from build123d import *

# Parameters (mm, degrees)
F0_W      = 60
F0_H      = 38
F1_DEPTH  = 2
F2_W      = 55.6
F2_H      = 33.6
F2_W_2    = 53.6
F2_H_2    = 31.6
F3_DEPTH  = 6
F4_W      = 45
F4_H      = 35
F5_DEPTH  = 1
F6_R      = 2
F7_R      = 1
F8_DEPTH  = 8.001
F9_R      = 1
F10_DEPTH = 35.801
F11_SIZE  = 1


with BuildPart() as f1:
    # F0 (on Top) → F1 (new body)
    with BuildSketch(Plane.XY):
        with Locations((30, -19)):
            Rectangle(F0_W, F0_H)
    extrude(amount=F1_DEPTH)

    # F2 (on face) → F3 (join)
    with BuildSketch(Plane.XY.offset(2)):
        with Locations((30, -19)):
            Rectangle(F2_W, F2_H)
        with Locations((30, -19)):
            Rectangle(F2_W_2, F2_H_2, mode=Mode.SUBTRACT)
    extrude(amount=F3_DEPTH)

    # F4 (on face) → F5 (cut)
    with BuildSketch(Plane(origin=(0, 0, 0), x_dir=(1, 0, 0), z_dir=(0, 0, -1))):
        with Locations((24.5, 19)):
            Rectangle(F4_W, F4_H)
    extrude(amount=-F5_DEPTH, mode=Mode.SUBTRACT)

    # F6
    f6_edges = [f1.edges().sort_by_distance(p)[0] for p in [
        (0, -38, 1),
        (0, 0, 1),
        (60, -38, 1),
        (60, 0, 1),
    ]]
    fillet(f6_edges, radius=F6_R)

    # F7 (on face) → F8 (cut, through all)
    with BuildSketch(Plane(origin=(0, 0, 0), x_dir=(1, 0, 0), z_dir=(0, 0, -1))):
        with Locations((9.5, 32.5)):
            Circle(F7_R)
        with Locations((39.5, 32.5)):
            Circle(F7_R)
    extrude(amount=-F8_DEPTH, mode=Mode.SUBTRACT)

    # F9 (on face) → F10 (cut, through all)
    with BuildSketch(Plane(origin=(0, -2.2, 0), x_dir=(-1, 0, 0), z_dir=(0, 1, 0))):
        with Locations((-54, 5)):
            Circle(F9_R)
        with Locations((-6, 5)):
            Circle(F9_R)
    extrude(amount=-F10_DEPTH, mode=Mode.SUBTRACT)

    # F11
    f11_edges = [f1.edges().sort_by_distance(p)[0] for p in [
        (2.2, -2.2, 5),
        (2.2, -35.8, 5),
        (57.8, -35.8, 5),
        (57.8, -2.2, 5),
    ]]
    chamfer(f11_edges, length=F11_SIZE)


solid = f1.part
Geometry: final body of the model. Coordinates: model frame, mm. A direction names the side the tool comes from. Coordinates: 2 decimals unless noted, no trailing zeros. Order: outer loops, then holes, each group sorted by start corner. A loop starts at its lowest first (then second) coordinate and runs counter-clockwise, first axis right, second up. Notation, with made-up numbers: (-16, -19) - (8, -19) arc R20 cw to (8, -12) - close; hole circle Ø10 at (14.25, 68.25). An arc over 180 degrees is marked (long way). Use one line per item in the form item = value.
1) Ray query, L1, parallel to Y at x = 34, z = 2.25; L2, parallel to X at y = -32, z = 3; L3, parallel to Z at x = 54, y = -35.1. Return the intervals inside material, ascending.
Solutions:
L1 = -35.8 to -34.8, -3.2 to -2.2
L2 = 2.2 to 3.2, 56.8 to 57.8
L3 = 0 to 4, 6 to 8
2) Section D-D (y = -32.5). Return loops of the section in (x, z).
Solutions:
outline = (0, 0) - (2, 0) - (2, 1) - (8.5, 1) - (8.5, 2) - (3.2, 2) - (3.2, 8) - (2.2, 8) - (2.2, 2) - (0, 2) - close; (10.5, 1) - (38.5, 1) - (38.5, 2) - (10.5, 2) - close; (40.5, 1) - (47, 1) - (47, 0) - (60, 0) - (60, 2) - (57.8, 2) - (57.8, 8) - (56.8, 8) - (56.8, 2) - (40.5, 2) - close
3) Pin query (flat end, axial travel): pin 1 (2.5 mm diameter, centred on x = 54, z = 5, fed in from +Y); pin 2 (1.8 mm diameter, centred on x = 30.5, z = 6.5, fed in from -Y); pin 3 (1.8 mm diameter, centred on y = -26.5, z = 5, fed in from +X). Return the tip coordinate at first contact, or that it passes through.
Solutions:
pin_1 = -2.2
pin_2 = -35.8
pin_3 = 57.8
4) Section B-B (x = 54). Return loops of the section in (y, z), then the cut area to 3 significant figures.
Solutions:
outline = (-38, 0) - (0, 0) - (0, 2) - (-2.2, 2) - (-2.2, 4) - (-3.2, 4) - (-3.2, 2) - (-34.8, 2) - (-34.8, 4) - (-35.8, 4) - (-35.8, 2) - (-38, 2) - close; (-35.8, 6) - (-34.8, 6) - (-34.8, 8) - (-35.8, 8) - close; (-3.2, 6) - (-2.2, 6) - (-2.2, 8) - (-3.2, 8) - close
area = 84.0 mm^2
5) Section A-A (z = 5). Return loops of the section in (x, y).
Solutions:
outline = (2.2, -34.8) - (3.2, -35.8) - (5, -35.8) - (5, -34.8) - (3.2, -34.8) - (3.2, -3.2) - (5, -3.2) - (5, -2.2) - (3.2, -2.2) - (2.2, -3.2) - close; (7, -35.8) - (53, -35.8) - (53, -34.8) - (7, -34.8) - close; (7, -3.2) - (53, -3.2) - (53, -2.2) - (7, -2.2) - close; (55, -35.8) - (56.8, -35.8) - (57.8, -34.8) - (57.8, -3.2) - (56.8, -2.2) - (55, -2.2) - (55, -3.2) - (56.8, -3.2) - (56.8, -34.8) - (55, -34.8) - close
6) Section C-C (y = -28). Return loops of the section in (x, z), then the cut area to 3 significant figures.
Solutions:
outline = (0, 0) - (2, 0) - (2, 1) - (47, 1) - (47, 0) - (60, 0) - (60, 2) - (57.8, 2) - (57.8, 8) - (56.8, 8) - (56.8, 2) - (3.2, 2) - (3.2, 8) - (2.2, 8) - (2.2, 2) - (0, 2) - close
area = 87.0 mm^2
7) Set-up query: faces 5 (the face through (24, -19, 1)), 6 (the face through (30, 0, 1)), 7 (the face through (30, -2.2, 5)), 8 (the face through (6.737, -2.693, 5.676)), 9 (the face through (30, -3.2, 5)). Return all of +Z, -Z, +X, -X, +Y, -Y with unobstructed straight access to the full face (end or side cutting, diameter ignored); none if empty.
Solutions:
face_5 = -Z
face_6 = +Z, -Z, +X, -X, +Y
face_7 = +Z, +X, -X, +Y
face_8 = +Y, -Y
face_9 = +Z
8) Mould query, pull axis X, two halves, no side actions, for faces 1 (the face through (55, -35, 5)), 2 (the face through (3.2, -19, 5)), 3 (the face through (57.8, -19, 5)), 4 (the face through (30, -35.8, 5)). Classes: +X half, -X half, draft (parallel to the pull), parting line (faces both ways), or undercut.
Solutions:
face_1 = undercut
face_2 = undercut
face_3 = +X half
face_4 = draft
